Job drawing, mm, ordinate dimensions from the low corner. One solid piece. Round coordinates to 2 decimals unless told otherwise and drop trailing zeros. Use CSV: the item, a comma, the result in double quotes.
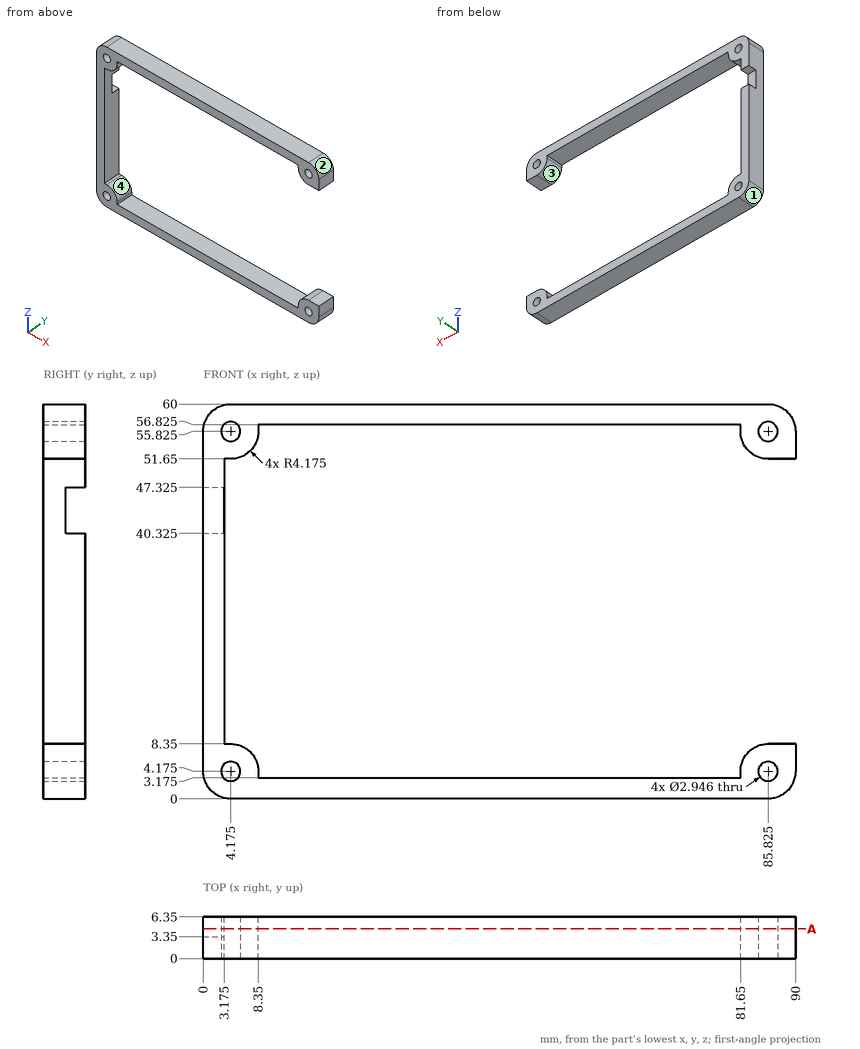
(1) Pull direction Z, two halves, no side cores. Call the marked faces 1, 2, 3 and 4: released by +Z, released by -Z, zero draft, split by the parting line, or undercut.
Reply:
face 1,"released by -Z"
face 2,"released by +Z"
face 3,"undercut"
face 4,"undercut"
(2) Drop flat-ended pins along their axis: P1, Ø2, axis at x = 87.5, y = 2.5, coming from the -Z side (1 decimal); P2, Ø0.9, axis at x = 1.5, y = 5, coming from the -Z side; P3, Ø2, axis at x = 11, y = 2, coming from the -Z side; P4, Ø0.8, axis at y = 2.5, z = 56.5, coming from the -X side. Give the stop position or say it passes through.
Reply:
P1,"z = 0.1"
P2,"z = 0.64"
P3,"z = 0"
P4,"x = 0.01"
(3) Probe probe 1 along Z at (x, y) = (80.5, 3.5) (1 decimal); probe 2 along X at (y, z) = (6, 57) (1 decimal); probe 3 along X at (y, z) = (6.25, 24.5) (1 decimal). List the from-to ranges inside material, lowest first. Write a range as [from, to].
Reply:
probe 1,"[0, 3.2], [56.8, 60]"
probe 2,"[0.2, 3.3], [5.1, 84.9], [86.7, 89.8]"
probe 3,"[0, 3.2]"
(4) Cut at A-A, the plane y = 4.5. State how many separate pieces and enclosed holes the cut face has.
Reply:
separate pieces,"2"
enclosed holes,"4"
